The model under review builds one solid part; all positions refer to its coordinate system, in mm. Face numbers are marked on the shaded views. Round coordinates to 2 decimals unless told otherwise and drop trailing zeros. Write each loop counter-clockwise with the first axis right and the second up, starting at its lowest first coordinate (ties: lowest second). Pieces come first, ordered by that corner, then holes. Notation, with made-up numbers: (46, -40) -> (89, -40) arc R8 cw to (89, -26) -> close; hole circle Ø2 at (54.25, -8.5). An arc over 180 degrees is marked (long way). Return JSON: item names as keys, results as strings. Group by question number.
1. Take a section at C-C, the plane z = 2.75. Write out the cut boundary in (x, y).
2. Clearance check with a flat-ended pin moving along its axis: P1, Ø3, axis at x = 0, y = 0, coming from the +Z side. State where the tip first meets the part, or that it passes through.
3. Take a section at A-A, the plane y = 0. Write out the cut boundary in (x, z), then the cut area to 3 significant figures.
4. Mouldability with a two-part tool opening along Y and no side actions: class the marked faces 1, 2 and 3 as pulls with the +Y half, pulls with the -Y half, needs draft (parallel to the pull), parting line crosses it, or undercut.
5. For line 1 along Y through (x, z) = (0, 3.1); line 2 along X through (y, z) = (0, 18.1); line 3 along X through (y, z) = (-0.8, 9.9), list the stretches that pass through material, from the lowest coordinate up. Write a range as from..to.
6. Take a section at B-B, the plane x = 0. Write out the cut boundary in (y, z).
7. Take a section at D-D, the plane y = -1.5. Write out the cut boundary in (x, z), then the cut area to 3 significant figures.
from build123d import *

# Parameters (mm, degrees)
F0_W          = 16.5
F0_H          = 6.5
F0_R          = 2
F1_DEPTH      = 19.4
F2_R          = 6.04
F3_DEPTH      = 25
F3_DEPTH_BACK = 25
F4_DEPTH      = 3
F5_R          = 2
F6_R          = 0.5


with BuildPart() as f1:
    # F0 (on Top) → F1 (new body)
    with BuildSketch(Plane.XY):
        Rectangle(F0_W, F0_H)
        Circle(F0_R, mode=Mode.SUBTRACT)
    extrude(amount=F1_DEPTH)

    # F2 (on face) → F3 (cut, two sides)
    with BuildSketch(Plane.XZ.offset(3.25)) as f3_sk:
        with Locations((0, 9.9)):
            Circle(F2_R)
    extrude(amount=-F3_DEPTH, mode=Mode.SUBTRACT)
    extrude(f3_sk.sketch, amount=-F3_DEPTH_BACK, mode=Mode.SUBTRACT)

    # F0 (on Top) → F4 (cut)
    with BuildSketch(Plane.XY):
        Rectangle(F0_W, F0_H)
        Circle(F0_R, mode=Mode.SUBTRACT)
    extrude(amount=-F4_DEPTH, mode=Mode.SUBTRACT)

    # F5
    f5_edges = [f1.edges().sort_by_distance(p)[0] for p in [
        (8.25, -3.25, 9.7),
        (-8.25, -3.25, 9.7),
        (-8.25, 3.25, 9.7),
        (8.25, 3.25, 9.7),
    ]]
    fillet(f5_edges, radius=F5_R)

    # F6
    f6_edges = [f1.edges().sort_by_distance(p)[0] for p in [
        (-6.04, -3.25, 9.9),
        (-6.04, 3.25, 9.9),
    ]]
    fillet(f6_edges, radius=F6_R)


solid = f1.part
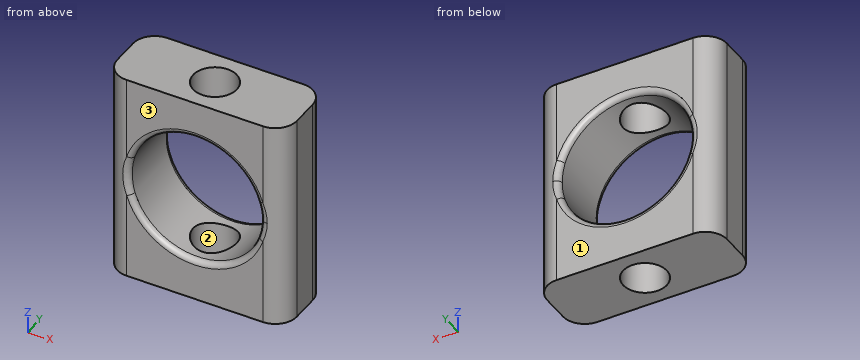
Output:
{
 "1": {"outline": "(-8.25, -1.25) arc R2 ccw to (-6.25, -3.25) -> (6.25, -3.25) arc R2 ccw to (8.25, -1.25) -> (8.25, 1.25) arc R2 ccw to (6.25, 3.25) -> (-6.25, 3.25) arc R2 ccw to (-8.25, 1.25) -> close; hole circle Ø4 at (0, 0)"},
 "2": {"P1": "passes through"},
 "3": {"outline": "(-8.25, 0) -> (-2, 0) -> (-2, 4.2) arc R6.04 cw to (-2, 15.6) -> (-2, 19.4) -> (-8.25, 19.4) -> close; (2, 0) -> (8.25, 0) -> (8.25, 19.4) -> (2, 19.4) -> (2, 15.6) arc R6.04 cw to (2, 4.2) -> close", "area": "175 mm^2"},
 "4": {"face 1": "pulls with the +Y half", "face 2": "undercut", "face 3": "pulls with the -Y half"},
 "5": {"line 1": "y = -3.25..-2, 2..3.25", "line 2": "x = -8.25..-2, 2..8.25", "line 3": "x = -8.25..-6.04, 6.04..8.25"},
 "6": {"outline": "(-3.25, 0) -> (-2, 0) -> (-2, 3.86) -> (-2.75, 3.86) arc R0.5 ccw to (-3.25, 3.36) -> close; (-3.25, 16.44) arc R0.5 ccw to (-2.75, 15.94) -> (-2, 15.94) -> (-2, 19.4) -> (-3.25, 19.4) -> close; (2, 0) -> (3.25, 0) -> (3.25, 3.36) arc R0.5 ccw to (2.75, 3.86) -> (2, 3.86) -> close; (2, 15.94) -> (2.75, 15.94) arc R0.5 ccw to (3.25, 16.44) -> (3.25, 19.4) -> (2, 19.4) -> close"},
 "7": {"outline": "(-8.23, 0) -> (-1.32, 0) -> (-1.32, 4.01) arc R6.04 cw to (-1.32, 15.79) -> (-1.32, 19.4) -> (-8.23, 19.4) -> close; (1.32, 0) -> (8.23, 0) -> (8.23, 19.4) -> (1.32, 19.4) -> (1.32, 15.79) arc R6.04 cw to (1.32, 4.01) -> close", "area": "185 mm^2"}
}
